Check sheet for the drawn part. Datum: minimum x, y, z corner. Units: mm. A direction names the side the tool comes from. Round coordinates to 2 decimals unless told otherwise and drop trailing zeros. Write each loop counter-clockwise with the first axis right and the second up, starting at its lowest first coordinate (ties: lowest second). Pieces come first, ordered by that corner, then holes. Notation, with made-up numbers: (47, 0.25) - (103, 0.25) arc R25 ccw to (103, 28.25) - close; hole circle Ø8 at (-4.5, 74.25). An arc over 180 degrees is marked (long way). Answer as a JSON object with one key per item and string values.
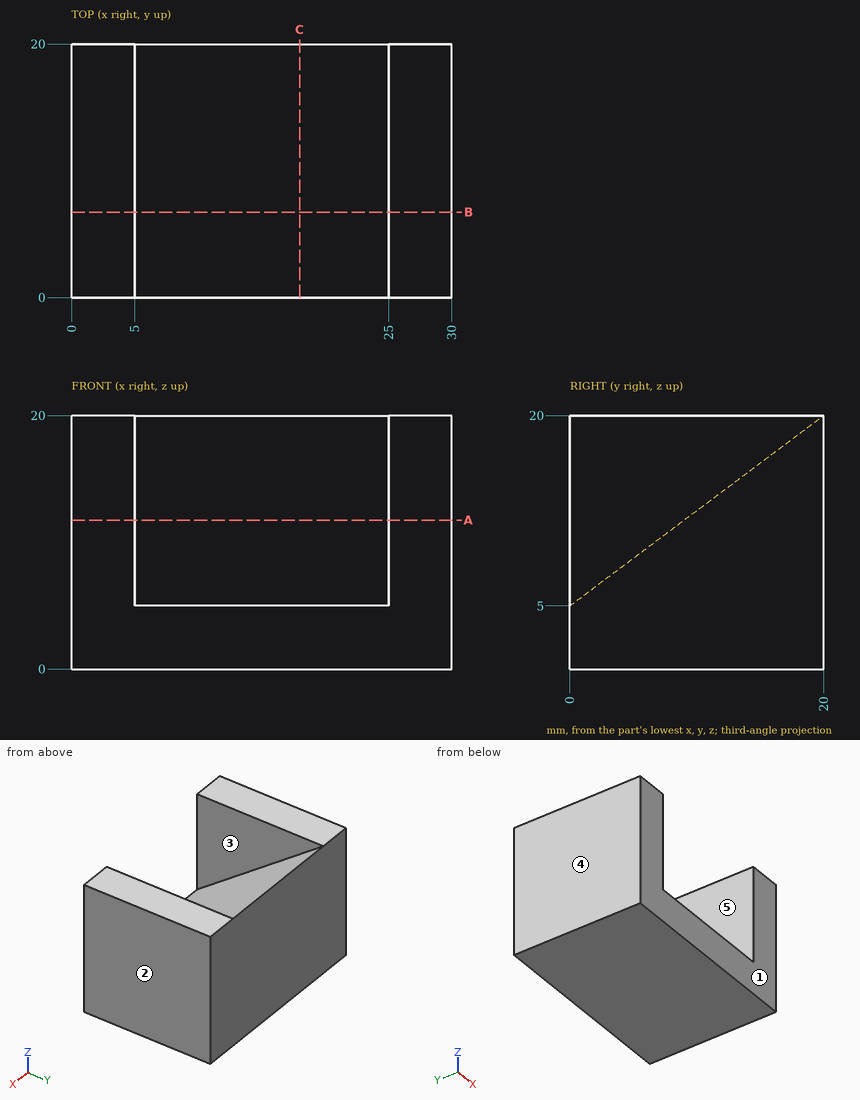
Q1. Section check A-A, the plane z = 11.75. Record the cut outline in (x, y).
Geometry check:
{"outline": "(0, 0) - (5, 0) - (5, 9) - (25, 9) - (25, 0) - (30, 0) - (30, 20) - (0, 20) - close"}
Q2. Gauge pin test, flat ends, axial feed: P1, Ø1, axis at x = 23, y = 10, coming from the +Z side (3 decimals); P2, Ø2, axis at x = 16, z = 18, coming from the -Y side. Record the tip position at first contact, or that the pin passes through.
Geometry check:
{"P1": "stops at z = 12.875", "P2": "stops at y = 16"}
Q3. Set-up check for the marked faces 4 and 5: record each of +Z, -Z, +X, -X, +Y, -Y from which the full face is reachable in a straight line by a thin tool's end or side.
Geometry check:
{"face 4": "+Z, -Z, -X, +Y, -Y", "face 5": "+Z, -Y"}
Q4. Material ranges on line 1 along X through (y, z) = (14.75, 18.5); line 2 along Z through (x, y) = (18.5, 14.5) (3 decimals); line 3 along Z through (x, y) = (10.5, 13.75), recorded low to high. Write a range as [from, to].
Geometry check:
{"line 1": "x = [0, 5], [25, 30]", "line 2": "z = [0, 15.875]", "line 3": "z = [0, 15.31]"}
Q5. Section check C-C, the plane x = 18. Record the cut outline in (y, z), then the cut area to 3 significant figures.
Geometry check:
{"outline": "(0, 0) - (20, 0) - (20, 20) - (0, 5) - close", "area": "250 mm2"}
Q6. Section check B-B, the plane y = 6.75. Record the cut outline in (x, z).
Geometry check:
{"outline": "(0, 0) - (30, 0) - (30, 20) - (25, 20) - (25, 10.06) - (5, 10.06) - (5, 20) - (0, 20) - close"}
Q7. Release check for a two-part mould opening along X. For the marked faces 1, 2 and 3 record: released by +X, released by -X, zero draft, split by the parting line, or undercut.
Geometry check:
{"face 1": "zero draft", "face 2": "released by +X", "face 3": "undercut"}
